Source: CAD feature listing. Evaluate the final solid. Frame: model axes, mm. Face numbers are marked on the shaded views. A direction names the side the tool comes from. Give positions to 0.01 mm unless a question says otherwise; leave off trailing zeros. Order: outer loops, then holes, each group sorted by start corner. A loop starts at its lowest first (then second) coordinate and runs counter-clockwise, first axis right, second up. Notation, with made-up numbers: (45.5, -0.5) - (93.5, -0.5) arc R11 cw to (93.5, 9.5) - close; hole circle Ø1 at (82, 56.5). An arc over 180 degrees is marked (long way). Use CSV: the item, a comma, the result in double quotes.
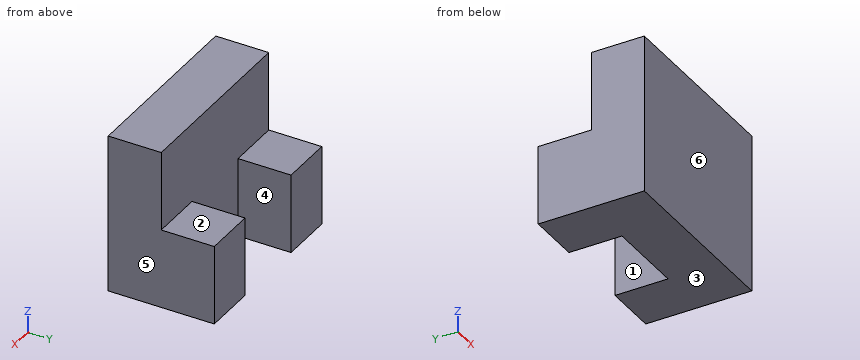
Autodesk Inventor part; units mm, degrees
ref_plane "YZ Plane" through (0, 0, 0) normal (1, 0, 0) x (0, 1, 0)
ref_plane "XZ Plane" through (0, 0, 0) normal (0, 1, 0) x (-1, 0, 0)
ref_plane "XY Plane" through (0, 0, 0) normal (0, 0, 1) x (1, 0, 0)
sketch "Sketch1" plane through (0, 0, 0) normal (0, 0, 1) x (1, 0, 0)
  line L0 (0, 12.7) -> (44.45, 12.7)
  line L1 (44.45, 12.7) -> (44.45, 0)
  line L2 (44.45, 0) -> (0, 0)
  line L3 (0, 0) -> (0, 12.7)
  dimension "d0" = 44.45
  dimension "d1" = 12.7
extrude "Extrusion1" add sketch "Sketch1" against normal blind 38.1
sketch "Sketch2" plane through (0, 12.7, 0) normal (0, 1, 0) x (1, 0, 0)
  line L0 (0, 0) -> (0, 38.1)
  line L1 (0, 38.1) -> (44.45, 38.1)
  line L2 (0, 19.05) -> (12.7, 19.05)
  line L3 (12.7, 19.05) -> (12.7, 38.1)
  line L4 (12.7, 38.1) -> (0, 38.1)
  line L5 (0, 38.1) -> (0, 19.05)
  line L6 (44.45, 0) -> (44.45, 38.1)
  line L7 (31.75, 38.1) -> (44.45, 38.1)
  line L8 (44.45, 38.1) -> (44.45, 19.05)
  line L9 (44.45, 19.05) -> (31.75, 19.05)
  line L10 (31.75, 19.05) -> (31.75, 38.1)
  dimension "d4" = 12.7
  dimension "d5" = 19.05
  dimension "d6" = 19.05
  dimension "d7" = 12.7
extrude "Extrusion2" add sketch "Sketch2" along normal blind 12.7
properties part number "A2.6_Titus_SktechSheetA4"
Item 1: Mould query, pull axis X, two halves, no side actions, for the marked faces 4, 5 and 6. Classes: released by +X, released by -X, zero draft, split by the parting line, or undercut.
Filled in:
face 4,"undercut"
face 5,"released by +X"
face 6,"zero draft"
Item 2: Section B-B on z = -34. Return the cut outline in (x, y).
Filled in:
outline,"(0, 0) - (44.45, 0) - (44.45, 25.4) - (31.75, 25.4) - (31.75, 12.7) - (12.7, 12.7) - (12.7, 25.4) - (0, 25.4) - close"
Item 3: Set-up query: the marked faces 1, 2 and 3. Return all of +Z, -Z, +X, -X, +Y, -Y with unobstructed straight access to the full face (end or side cutting, diameter ignored); none if empty.
Filled in:
face 1,"+Z, -Z, +Y"
face 2,"+Z, +X, -X, +Y"
face 3,"-Z, +X, -X, +Y, -Y"
Item 4: Section C-C on x = 40. Return the cut outline in (y, z).
Filled in:
outline,"(0, -38.1) - (25.4, -38.1) - (25.4, -19.05) - (12.7, -19.05) - (12.7, 0) - (0, 0) - close"
Item 5: Material intervals for line 1 (Y direction, x = 33.5, z = -18.5); line 2 (X direction, y = 15.25, z = -31.5); line 3 (Z direction, x = 2, y = 18.25), sorted ascending. Write a range as from..to.
Filled in:
line 1,"y = 0..12.7"
line 2,"x = 0..12.7, 31.75..44.45"
line 3,"z = -38.1..-19.05"
Item 6: First-contact query: pin 1 (6.5 mm diameter, centred on x = 4, y = 17.5, fed in from +Z). Flat tip, straight axial feed; report the tip coordinate or a pass-through.
Filled in:
pin 1,"stops at z = -19.05"
Item 7: Section D-D on x = 22.5. Return the cut outline in (y, z), then the cut area to 3 significant figures.
Filled in:
outline,"(0, -38.1) - (12.7, -38.1) - (12.7, 0) - (0, 0) - close"
area,"484 mm2"
Item 8: Section A-A on y = 16.5. Return the cut outline in (x, z), then the cut area to 3 significant figures.
Filled in:
outline,"(0, -38.1) - (12.7, -38.1) - (12.7, -19.05) - (0, -19.05) - close; (31.75, -38.1) - (44.45, -38.1) - (44.45, -19.05) - (31.75, -19.05) - close"
area,"484 mm2"
